The drawing under review shows one solid part. Ordinate dimensions are in mm from its lowest x, y, z. A direction names the side the tool comes from. Coordinates: 2 decimals unless noted, no trailing zeros. Write each loop counter-clockwise with the first axis right and the second up, starting at its lowest first coordinate (ties: lowest second). Pieces come first, ordered by that corner, then holes. Notation, with made-up numbers: (-23, 72.25) - (35, 72.25) arc R20 ccw to (35, 107.25) - close; hole circle Ø3 at (28, 62.5). An arc over 180 degrees is marked (long way). Use a Markdown table: item, result.
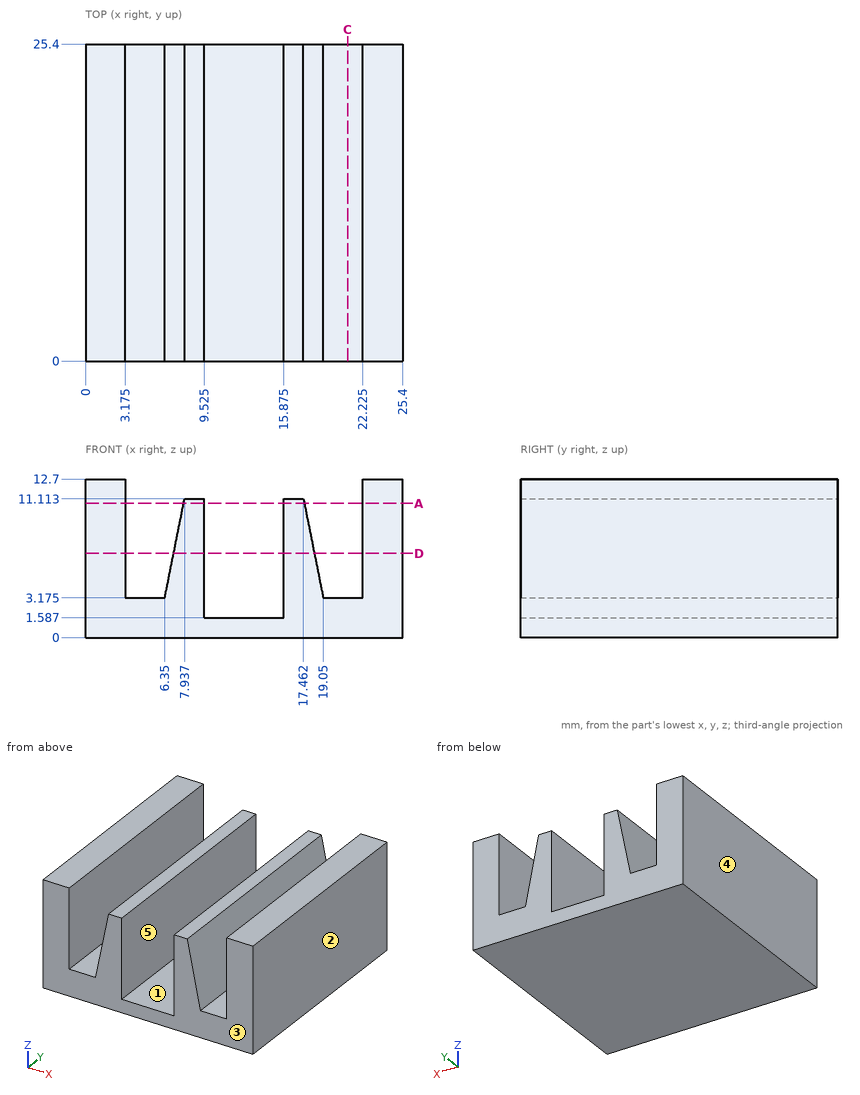
(1) Take a section at C-C on x = 21. Write out the cut boundary in (y, z) (1 decimal).
Determined:
| item | result |
|---|---|
| outline | (0, 0) - (25.4, 0) - (25.4, 3.2) - (0, 3.2) - close |
(2) Draft analysis for pull direction X (two halves, no side actions). For the marked faces 1, 2 and 3, state which applies: +X half, -X half, draft (parallel to the pull), parting line (faces both ways), or undercut.
Determined:
| item | result |
|---|---|
| face 1 | undercut |
| face 2 | +X half |
| face 3 | draft |
(3) For L1, parallel to X at y = 7.25, z = 11 (1 decimal); L2, parallel to X at y = 7.5, z = 10.5 (1 decimal); L3, parallel to X at y = 16.25, z = 1.75 (1 decimal), list the stretches that pass through material, from the lowest coordinate up. Write a range as from..to.
Determined:
| item | result |
|---|---|
| L1 | 0..3.2, 7.9..9.5, 15.9..17.5, 22.2..25.4 |
| L2 | 0..3.2, 7.8..9.5, 15.9..17.6, 22.2..25.4 |
| L3 | 0..9.5, 15.9..25.4 |
(4) Take a section at A-A on z = 10.75. Write out the cut boundary in (x, y) (1 decimal).
Determined:
| item | result |
|---|---|
| outline | (0, 0) - (3.2, 0) - (3.2, 25.4) - (0, 25.4) - close; (7.9, 0) - (9.5, 0) - (9.5, 25.4) - (7.9, 25.4) - close; (15.9, 0) - (17.5, 0) - (17.5, 25.4) - (15.9, 25.4) - close; (22.2, 0) - (25.4, 0) - (25.4, 25.4) - (22.2, 25.4) - close |
(5) For pin 1 (0.5 mm diameter, centred on x = 17, y = 7, fed in from +Z); pin 2 (3.5 mm diameter, centred on x = 4.5, y = 8.5, fed in from +Z); pin 3 (3 mm diameter, centred on x = 14, y = 11.5, fed in from +Z); pin 4 (1 mm diameter, centred on x = 20.5, y = 3.5, fed in from +Z) (1 decimal), all flat-tipped, find the tip position at first contact; note any pin that passes through.
Determined:
| item | result |
|---|---|
| pin 1 | z = 11.11 |
| pin 2 | z = 12.7 |
| pin 3 | z = 1.59 |
| pin 4 | z = 3.2 |
(6) Take a section at D-D on z = 6.75. Write out the cut boundary in (x, y) (1 decimal).
Determined:
| item | result |
|---|---|
| outline | (0, 0) - (3.2, 0) - (3.2, 25.4) - (0, 25.4) - close; (7.1, 0) - (9.5, 0) - (9.5, 25.4) - (7.1, 25.4) - close; (15.9, 0) - (18.3, 0) - (18.3, 25.4) - (15.9, 25.4) - close; (22.2, 0) - (25.4, 0) - (25.4, 25.4) - (22.2, 25.4) - close |
(7) Machinability: for the marked faces 4 and 5, which of the approach directions +Z, -Z, +X, -X, +Y, -Y give a long, thin tool a straight path to every point of the face, cutting with its end or side? Answer none if there is none.
Determined:
| item | result |
|---|---|
| face 4 | +Z, -Z, -X, +Y, -Y |
| face 5 | +Z, +Y, -Y |
